from build123d import *

# Parameters (mm, degrees)
SKETCH_1_W                        = 601
SKETCH_1_H                        = 306
SKETCH_1_R                        = 30
SM_BASE_FLANGE_1_DEPTH            = 1
SM_EDGE_FLANGE_1_STRIP_W          = 5.4732
SM_EDGE_FLANGE_1_STRIP_H          = 1
SM_EDGE_FLANGE_1_STRIP_CUT_DEPTH  = 501
SM_EDGE_FLANGE_1_RELIEF_W         = 5.9732
SM_EDGE_FLANGE_1_RELIEF_H         = 0.5
SM_EDGE_FLANGE_1_RELIEF_CUT_DEPTH = 1
SM_EDGE_FLANGE_1_DEPTH            = 501
SM_EDGE_FLANGE_2_STRIP_W          = 5.4732
SM_EDGE_FLANGE_2_STRIP_H          = 1
SM_EDGE_FLANGE_2_STRIP_CUT_DEPTH  = 206
SM_EDGE_FLANGE_2_RELIEF_W         = 5.9732
SM_EDGE_FLANGE_2_RELIEF_H         = 0.5
SM_EDGE_FLANGE_2_RELIEF_CUT_DEPTH = 1
SM_EDGE_FLANGE_2_DEPTH            = 206
SM_EDGE_FLANGE_3_STRIP_W          = 5.4732
SM_EDGE_FLANGE_3_STRIP_H          = 1
SM_EDGE_FLANGE_3_STRIP_CUT_DEPTH  = 501
SM_EDGE_FLANGE_3_RELIEF_W         = 5.9732
SM_EDGE_FLANGE_3_RELIEF_H         = 0.5
SM_EDGE_FLANGE_3_RELIEF_CUT_DEPTH = 1
SM_EDGE_FLANGE_3_DEPTH            = 501
SM_EDGE_FLANGE_4_STRIP_W          = 5.4732
SM_EDGE_FLANGE_4_STRIP_H          = 1
SM_EDGE_FLANGE_4_STRIP_CUT_DEPTH  = 206
SM_EDGE_FLANGE_4_RELIEF_W         = 5.9732
SM_EDGE_FLANGE_4_RELIEF_H         = 0.5
SM_EDGE_FLANGE_4_RELIEF_CUT_DEPTH = 1
SM_EDGE_FLANGE_4_DEPTH            = 206
SKETCH_15_R                       = 3
CUT_EXTRUDE_1_DEPTH               = 338.800606867


# Sheet-metal steps are written as plain solids
with BuildPart() as part:
    # Sketch 1 → 基体-法兰1 (new body)
    with BuildSketch(Plane.XY):
        Rectangle(SKETCH_1_W, SKETCH_1_H)
        with Locations((-195, 73)):
            Circle(SKETCH_1_R, mode=Mode.SUBTRACT)
    extrude(amount=-SM_BASE_FLANGE_1_DEPTH)

    # 边线-法兰1 strip (across the edge) → 边线-法兰1 strip cut (cut)
    with BuildSketch(Plane(origin=(-250.5, 153, -1), x_dir=(0, -1, 0), z_dir=(1, 0, 0))):
        with Locations((-1, -0.5)):
            Rectangle(SM_EDGE_FLANGE_1_STRIP_W, SM_EDGE_FLANGE_1_STRIP_H)
    extrude(amount=SM_EDGE_FLANGE_1_STRIP_CUT_DEPTH, mode=Mode.SUBTRACT)

    # 边线-法兰1 relief (on the sheet) → 边线-法兰1 relief cut (cut)
    with BuildSketch(Plane(origin=(-250.5, 151.2634, -1), x_dir=(0, -1, 0), z_dir=(0, 0, -1))):
        with Locations((-2.4866, 0.25)):
            Rectangle(SM_EDGE_FLANGE_1_RELIEF_W, SM_EDGE_FLANGE_1_RELIEF_H)
        with Locations((-2.4866, -501.25)):
            Rectangle(SM_EDGE_FLANGE_1_RELIEF_W, SM_EDGE_FLANGE_1_RELIEF_H)
    extrude(amount=-SM_EDGE_FLANGE_1_RELIEF_CUT_DEPTH, mode=Mode.SUBTRACT)

    # 边线-法兰1 section (across the edge) → 边线-法兰1 (add)
    with BuildSketch(Plane(origin=(-250.5, 153, -1), x_dir=(0, -1, 0), z_dir=(1, 0, 0))):
        with BuildLine():
            Line((0, 0.7366), (0, 19))
            Line((0, 19), (1, 19))
            Line((1, 19), (1, 0.7366))
            ThreePointArc((1, 0.7366), (1.215745145, 0.215745145), (1.7366, 0))
            Line((1.7366, 0), (1.7366, -1))
            ThreePointArc((1.7366, -1), (0.508638364, -0.491361636), (0, 0.7366))
        make_face()
    extrude(amount=SM_EDGE_FLANGE_1_DEPTH)

    # 边线-法兰2 strip (across the edge) → 边线-法兰2 strip cut (cut)
    with BuildSketch(Plane(origin=(300.5, 103, -1), x_dir=(-1, 0, 0), z_dir=(0, -1, 0))):
        with Locations((-1, -0.5)):
            Rectangle(SM_EDGE_FLANGE_2_STRIP_W, SM_EDGE_FLANGE_2_STRIP_H)
    extrude(amount=SM_EDGE_FLANGE_2_STRIP_CUT_DEPTH, mode=Mode.SUBTRACT)

    # 边线-法兰2 relief (on the sheet) → 边线-法兰2 relief cut (cut)
    with BuildSketch(Plane(origin=(298.7634, 103, -1), x_dir=(-1, 0, 0), z_dir=(0, 0, -1))):
        with Locations((-2.4866, 0.25)):
            Rectangle(SM_EDGE_FLANGE_2_RELIEF_W, SM_EDGE_FLANGE_2_RELIEF_H)
        with Locations((-2.4866, -206.25)):
            Rectangle(SM_EDGE_FLANGE_2_RELIEF_W, SM_EDGE_FLANGE_2_RELIEF_H)
    extrude(amount=-SM_EDGE_FLANGE_2_RELIEF_CUT_DEPTH, mode=Mode.SUBTRACT)

    # 边线-法兰2 section (across the edge) → 边线-法兰2 (add)
    with BuildSketch(Plane(origin=(300.5, 103, -1), x_dir=(-1, 0, 0), z_dir=(0, -1, 0))):
        with BuildLine():
            Line((0, 0.7366), (0, 19))
            Line((0, 19), (1, 19))
            Line((1, 19), (1, 0.7366))
            ThreePointArc((1, 0.7366), (1.215745145, 0.215745145), (1.7366, 0))
            Line((1.7366, 0), (1.7366, -1))
            ThreePointArc((1.7366, -1), (0.508638364, -0.491361636), (0, 0.7366))
        make_face()
    extrude(amount=SM_EDGE_FLANGE_2_DEPTH)

    # 边线-法兰3 strip (across the edge) → 边线-法兰3 strip cut (cut)
    with BuildSketch(Plane(origin=(250.5, -153, -1), x_dir=(0, 1, 0), z_dir=(-1, 0, 0))):
        with Locations((-1, -0.5)):
            Rectangle(SM_EDGE_FLANGE_3_STRIP_W, SM_EDGE_FLANGE_3_STRIP_H)
    extrude(amount=SM_EDGE_FLANGE_3_STRIP_CUT_DEPTH, mode=Mode.SUBTRACT)

    # 边线-法兰3 relief (on the sheet) → 边线-法兰3 relief cut (cut)
    with BuildSketch(Plane(origin=(250.5, -151.2634, -1), x_dir=(0, 1, 0), z_dir=(0, 0, -1))):
        with Locations((-2.4866, 0.25)):
            Rectangle(SM_EDGE_FLANGE_3_RELIEF_W, SM_EDGE_FLANGE_3_RELIEF_H)
        with Locations((-2.4866, -501.25)):
            Rectangle(SM_EDGE_FLANGE_3_RELIEF_W, SM_EDGE_FLANGE_3_RELIEF_H)
    extrude(amount=-SM_EDGE_FLANGE_3_RELIEF_CUT_DEPTH, mode=Mode.SUBTRACT)

    # 边线-法兰3 section (across the edge) → 边线-法兰3 (add)
    with BuildSketch(Plane(origin=(250.5, -153, -1), x_dir=(0, 1, 0), z_dir=(-1, 0, 0))):
        with BuildLine():
            Line((0, 0.7366), (0, 19))
            Line((0, 19), (1, 19))
            Line((1, 19), (1, 0.7366))
            ThreePointArc((1, 0.7366), (1.215745145, 0.215745145), (1.7366, 0))
            Line((1.7366, 0), (1.7366, -1))
            ThreePointArc((1.7366, -1), (0.508638364, -0.491361636), (0, 0.7366))
        make_face()
    extrude(amount=SM_EDGE_FLANGE_3_DEPTH)

    # 边线-法兰4 strip (across the edge) → 边线-法兰4 strip cut (cut)
    with BuildSketch(Plane(origin=(-300.5, -103, -1), x_dir=(1, 0, 0), z_dir=(0, 1, 0))):
        with Locations((-1, -0.5)):
            Rectangle(SM_EDGE_FLANGE_4_STRIP_W, SM_EDGE_FLANGE_4_STRIP_H)
    extrude(amount=SM_EDGE_FLANGE_4_STRIP_CUT_DEPTH, mode=Mode.SUBTRACT)

    # 边线-法兰4 relief (on the sheet) → 边线-法兰4 relief cut (cut)
    with BuildSketch(Plane(origin=(-298.7634, -103, -1), x_dir=(1, 0, 0), z_dir=(0, 0, -1))):
        with Locations((-2.4866, 0.25)):
            Rectangle(SM_EDGE_FLANGE_4_RELIEF_W, SM_EDGE_FLANGE_4_RELIEF_H)
        with Locations((-2.4866, -206.25)):
            Rectangle(SM_EDGE_FLANGE_4_RELIEF_W, SM_EDGE_FLANGE_4_RELIEF_H)
    extrude(amount=-SM_EDGE_FLANGE_4_RELIEF_CUT_DEPTH, mode=Mode.SUBTRACT)

    # 边线-法兰4 section (across the edge) → 边线-法兰4 (add)
    with BuildSketch(Plane(origin=(-300.5, -103, -1), x_dir=(1, 0, 0), z_dir=(0, 1, 0))):
        with BuildLine():
            Line((0, 0.7366), (0, 19))
            Line((0, 19), (1, 19))
            Line((1, 19), (1, 0.7366))
            ThreePointArc((1, 0.7366), (1.215745145, 0.215745145), (1.7366, 0))
            Line((1.7366, 0), (1.7366, -1))
            ThreePointArc((1.7366, -1), (0.508638364, -0.491361636), (0, 0.7366))
        make_face()
    extrude(amount=SM_EDGE_FLANGE_4_DEPTH)

    # 草图15 → 切除-拉伸1 (cut, through all)
    with BuildSketch(Plane.XY):
        with Locations((-291, -144)):
            Circle(SKETCH_15_R)
        with Locations((-291, 143)):
            Circle(SKETCH_15_R)
        with Locations((291, 143)):
            Circle(SKETCH_15_R)
        with Locations((291, -144)):
            Circle(SKETCH_15_R)
    extrude(amount=-CUT_EXTRUDE_1_DEPTH, mode=Mode.SUBTRACT)


solid = part.part
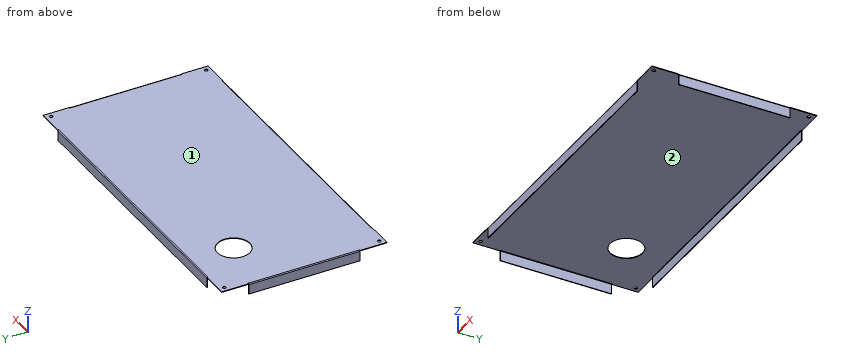
Read the model definition and answer for the solid it produces. Units are mm, in the model's axes. Face numbers are marked on the shaded views. Round coordinates to 2 decimals unless told otherwise and drop trailing zeros. Loops run counter-clockwise (first coordinate to the right, second up) from the corner with the lowest first, then second, coordinate; pieces in that order, holes last.
Q1. Section B-B on y = 73 is taken. Write down the section's boundary in (x, z).
Q2. Each of these flat-tipped pins is pushed along its axis until it touches: pin 1 (2.5 mm diameter, centred on x = 300, z = -10.5, fed in from -Y); pin 2 (12 mm diameter, centred on x = -183.5, y = 9, fed in from -Z); pin 3 (1.1 mm diameter, centred on x = -300, z = -8, fed in from +Y). Where does it stop, or does it pass through?
Q3. Section C-C on x = 228 is taken. Write down the section's boundary in (y, z), and give its area (3 significant figures).
Q4. Section D-D on y = -48.5 is taken. Write down the section's boundary in (x, z).
Q5. Determine the mould class of the marked faces 1 and 2 for opening direction X: released by +X, released by -X, zero draft, split by the parting line, or undercut.
Q6. Consider probe 1 along Y at (x, z) = (291, -0.25); probe 2 along X at (y, z) = (-29, -10); probe 3 along Y at (x, z) = (-168, -17). Determine where each line is inside the solid, lowest interval first.
Q7. Section A-A on z = -10.25 is taken. Write down the section's boundary in (x, y), and give its area (3 significant figures).
Output:
1. outline: (-300.5, -20) - (-299.5, -20) - (-299.5, -1.74) arc R0.74 cw to (-298.76, -1) - (-225, -1) - (-225, 0) - (-298.76, 0) arc R1.74 ccw to (-300.5, -1.74) - close; (-165, -1) - (298.76, -1) arc R0.74 cw to (299.5, -1.74) - (299.5, -20) - (300.5, -20) - (300.5, -1.74) arc R1.74 ccw to (298.76, 0) - (-165, 0) - close
2. pin 1: stops at y = -103
2. pin 2: stops at z = -1
2. pin 3: stops at y = 103
3. outline: (-153, -20) - (-152, -20) - (-152, -1.74) arc R0.74 cw to (-151.26, -1) - (151.26, -1) arc R0.74 cw to (152, -1.74) - (152, -20) - (153, -20) - (153, -1.74) arc R1.74 ccw to (151.26, 0) - (-151.26, 0) arc R1.74 ccw to (-153, -1.74) - close
3. area: 343 mm2
4. outline: (-300.5, -20) - (-299.5, -20) - (-299.5, -1.74) arc R0.74 cw to (-298.76, -1) - (298.76, -1) arc R0.74 cw to (299.5, -1.74) - (299.5, -20) - (300.5, -20) - (300.5, -1.74) arc R1.74 ccw to (298.76, 0) - (-298.76, 0) arc R1.74 ccw to (-300.5, -1.74) - close
5. face 1: zero draft
5. face 2: undercut
6. probe 1: y = -153 to -147, -141 to 140, 146 to 153
6. probe 2: x = -300.5 to -299.5, 299.5 to 300.5
6. probe 3: y = -153 to -152, 152 to 153
7. outline: (-300.5, -103) - (-299.5, -103) - (-299.5, 103) - (-300.5, 103) - close; (-250.5, -153) - (250.5, -153) - (250.5, -152) - (-250.5, -152) - close; (-250.5, 152) - (250.5, 152) - (250.5, 153) - (-250.5, 153) - close; (299.5, -103) - (300.5, -103) - (300.5, 103) - (299.5, 103) - close
7. area: 1,410 mm2
